Here's how the part is built. I have some questions about the finished solid (model axes, mm). Face numbers are marked on the shaded views. A direction names the side the tool comes from. Give positions to 0.01 mm unless a question says otherwise; leave off trailing zeros. Loops run counter-clockwise (first coordinate to the right, second up) from the corner with the lowest first, then second, coordinate; pieces in that order, holes last.
Q1. I need wall thicknesses on line 1 (Y direction, x = -3, z = -21.5); line 2 (Y direction, x = -1.5, z = -14); line 3 (Z direction, x = -1.25, y = 25). Which ranges of each line are inside material? Lowest first, please.
Q2. We'd pull the mould along Y, two halves only. Please class the marked faces 1, 2 and 3: +Y half, -Y half, draft (parallel to the pull), parting line (faces both ways), or undercut.
Q3. If we section it at A-A (z = -21): Please give me the cut outline in (x, y), plus the area to 3 significant figures.
Q4. Will these pins go through, and if not, where does the flat tip stop? P1, Ø1.5, axis at x = 1, y = 7.5, coming from the -Z side; P2, Ø2, axis at x = 0, z = -16.5, coming from the -Y side.
Q5. For the marked faces 4 and 5, which set-ups out of +Z, -Z, +X, -X, +Y, -Y let a thin tool reach every point of the face, with its end or its side?
Q6. If we section it at C-C (z = -14): Please give me the cut outline in (x, y), plus the area to 3 significant figures.
Q7. If we section it at D-D (y = -12.5): Please give me the cut outline in (x, z).
from build123d import *

# Parameters (mm, degrees)
F0_W     = 7
F0_H     = 70
F1_DEPTH = 5
F2_W     = 7
F2_H     = 3
F3_DEPTH = 26
F4_W     = 7
F4_H     = 8.6
F5_DEPTH = 3
F6_W     = 7
F6_H     = 3
F7_DEPTH = 18
F8_W     = 7
F8_H     = 9
F9_DEPTH = 1.6
F10_SIZE = 4
F11_SIZE = 1.59999


# Not quite as in the source:
# - a fillet or chamfer is up to 0.001 mm smaller than in the source, because OpenCascade refuses the exact size


with BuildPart() as f1:
    # F0 (on Top) → F1 (new body)
    with BuildSketch(Plane.XY):
        Rectangle(F0_W, F0_H)
    extrude(amount=F1_DEPTH)

    # F2 (on face) → F3 (join)
    with BuildSketch(Plane(origin=(0, 0, 0), x_dir=(1, 0, 0), z_dir=(0, 0, -1))):
        with Locations((0, -33.5)):
            Rectangle(F2_W, F2_H)
    extrude(amount=F3_DEPTH)

    # F4 (on face) → F5 (join)
    with BuildSketch(Plane(origin=(0, 0, -26), x_dir=(1, 0, 0), z_dir=(0, 0, -1))):
        with Locations((0, -30.7)):
            Rectangle(F4_W, F4_H)
    extrude(amount=F5_DEPTH)

    # F6 (on face) → F7 (join)
    with BuildSketch(Plane.XY.offset(-26)):
        with Locations((0, 27.9)):
            Rectangle(F6_W, F6_H)
    extrude(amount=F7_DEPTH)

    # F8 (on face) → F9 (join)
    with BuildSketch(Plane(origin=(0, 29.4, 0), x_dir=(-1, 0, 0), z_dir=(0, 1, 0))):
        with Locations((0, -12.5)):
            Rectangle(F8_W, F8_H)
    extrude(amount=F9_DEPTH)

    # F10
    f10_edges = [f1.edges().sort_by_distance(p)[0] for p in [
        (0, 31, -8),
    ]]
    chamfer(f10_edges, length=F10_SIZE)

    # F11 (size 1.6 in the source; OpenCascade refuses exactly that, so slightly less here)
    f11_edges = [f1.edges().sort_by_distance(p)[0] for p in [
        (0, 31, -17),
    ]]
    chamfer(f11_edges, length=F11_SIZE)


solid = f1.part
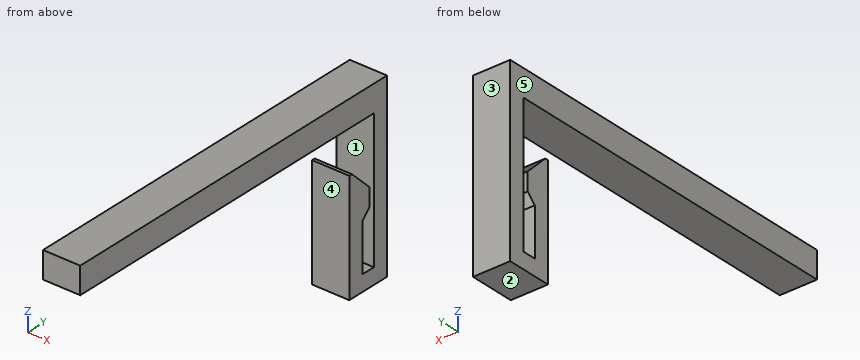
Check sheet entries:
1. line 1: y = 26.4 to 29.4, 32 to 35
1. line 2: y = 26.4 to 31, 32 to 35
1. line 3: z = 0 to 5
2. face 1: undercut
2. face 2: draft
2. face 3: +Y half
3. outline: (-3.5, 26.4) - (3.5, 26.4) - (3.5, 29.4) - (-3.5, 29.4) - close; (-3.5, 32) - (3.5, 32) - (3.5, 35) - (-3.5, 35) - close
3. area: 42.0 mm2
4. P1: stops at z = 0
4. P2: stops at y = 26.4
5. face 4: -Z, +X, -X, -Y
5. face 5: +Z, -Z, -X, +Y, -Y
6. outline: (-3.5, 26.4) - (3.5, 26.4) - (3.5, 31) - (-3.5, 31) - close; (-3.5, 32) - (3.5, 32) - (3.5, 35) - (-3.5, 35) - close
6. area: 53.2 mm2
7. outline: (-3.5, 0) - (3.5, 0) - (3.5, 5) - (-3.5, 5) - close
